Here's how the part is built. I have some questions about the finished solid (model axes, mm). Face numbers are marked on the shaded views. A direction names the side the tool comes from. Round coordinates to 2 decimals unless told otherwise and drop trailing zeros. Order: outer loops, then holes, each group sorted by start corner. A loop starts at its lowest first (then second) coordinate and runs counter-clockwise, first axis right, second up.
```python
from build123d import *

# Parameters (mm, degrees)
BOSS_EXTRUDE1_DEPTH             = 10
SKETCH5_W                       = 22
SKETCH5_H                       = 7
CUT_EXTRUDE2_DEPTH              = 28.349588662
FILLET3_R                       = 0.5
M3X0_5_TAPPED_HOLE1_D           = 2.5
M3X0_5_TAPPED_HOLE1_CSINK_D     = 3.05
M3X0_5_TAPPED_HOLE1_CSINK_ANGLE = 90
M8X1_0_TAPPED_HOLE1_D           = 7
M8X1_0_TAPPED_HOLE1_CSINK_D     = 8.05
M8X1_0_TAPPED_HOLE1_CSINK_ANGLE = 90


with BuildPart() as part:
    # Sketch1 → Boss-Extrude1 (new body)
    with BuildSketch(Plane.XY):
        with BuildLine():
            Line((-14, 9.141740125), (14, 9.141740125))
            ThreePointArc((14, 9.141740125), (16.828427125, 7.97016725), (18, 5.141740125))
            Line((18, 5.141740125), (18, -4.858259875))
            ThreePointArc((18, -4.858259875), (16.828427125, -7.686686999), (14, -8.858259875))
            Line((14, -8.858259875), (-14, -8.858259875))
            ThreePointArc((-14, -8.858259875), (-16.828427125, -7.686686999), (-18, -4.858259875))
            Line((-18, -4.858259875), (-18, 5.141740125))
            ThreePointArc((-18, 5.141740125), (-16.828427125, 7.97016725), (-14, 9.141740125))
        make_face()
    extrude(amount=BOSS_EXTRUDE1_DEPTH)

    # Sketch5 → Cut-Extrude2 (cut, through all)
    with BuildSketch(Plane(origin=(0, 9.141740125, 0), x_dir=(1, 0, 0), z_dir=(0, 1, 0))):
        Rectangle(SKETCH5_W, SKETCH5_H)
    extrude(amount=-CUT_EXTRUDE2_DEPTH, mode=Mode.SUBTRACT)

    # Fillet3
    fillet3_edges = [part.edges().sort_by_distance(p)[0] for p in [
        (-16.828427125, 7.97016725, 10),
        (-18, 0.141740125, 10),
        (-16.828427125, -7.686686999, 10),
        (0, -8.858259875, 10),
        (16.828427125, -7.686686999, 10),
        (11, -8.858259875, 1.75),
        (18, 0.141740125, 10),
        (0, -8.858259875, 3.5),
        (11, 0.141740125, 3.5),
        (-11, -8.858259875, 1.75),
        (-11, 0.141740125, 3.5),
        (-11, 9.141740125, 1.75),
        (0, 9.141740125, 3.5),
        (11, 9.141740125, 1.75),
        (16.828427125, 7.97016725, 10),
        (0, 9.141740125, 10),
    ]]
    fillet(fillet3_edges, radius=FILLET3_R)

    # M3x0.5 Tapped Hole1 (through all)
    with Locations(Plane(origin=(-13.335, 0.141740125, 10), x_dir=(1, 0, 0), z_dir=(0, 0, 1))):
        with Locations((0, 0), (26.67, 0)):
            CounterSinkHole(M3X0_5_TAPPED_HOLE1_D / 2, M3X0_5_TAPPED_HOLE1_CSINK_D / 2, counter_sink_angle=M3X0_5_TAPPED_HOLE1_CSINK_ANGLE)

    # M8x1.0 Tapped Hole1 (through all)
    with Locations(Plane(origin=(0, 0.141740125, 10), x_dir=(1, 0, 0), z_dir=(0, 0, 1))):
        with Locations((0, 0)):
            CounterSinkHole(M8X1_0_TAPPED_HOLE1_D / 2, M8X1_0_TAPPED_HOLE1_CSINK_D / 2, counter_sink_angle=M8X1_0_TAPPED_HOLE1_CSINK_ANGLE)


solid = part.part
```
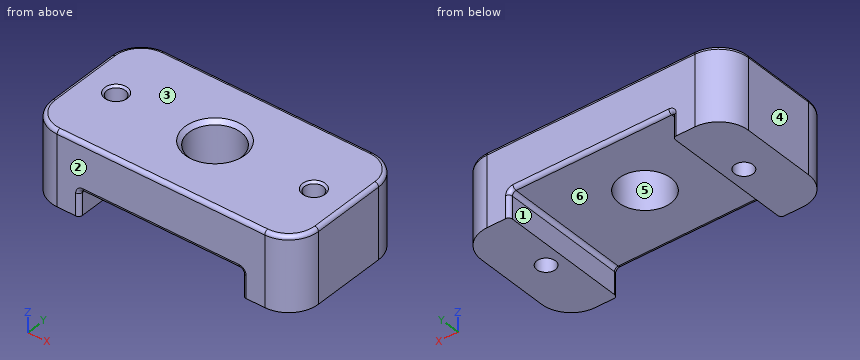
1) We'd pull the mould along X, two halves only. Please class the marked faces 3, 4, 5 and 6: +X half, -X half, draft (parallel to the pull), parting line (faces both ways), or undercut.
2) I'm going to push flat-ended pins straight in: pin 1 (4 mm diameter, centred on x = -2, z = 3, fed in from -Y); pin 2 (4 mm diameter, centred on x = 6.5, y = 7, fed in from -Z); pin 3 (3 mm diameter, centred on y = -7, z = 2.5, fed in from -X); pin 4 (2 mm diameter, centred on y = -6, z = 6, fed in from +X). Where does each tip first touch, or does it pass through?
3) If we section it at B-B (z = 1.5): Write out the boundary of the cut face in (x, y) (3 decimals).
4) I need wall thicknesses on line 1 (X direction, y = 0.25, z = 4.75); line 2 (Y direction, x = 0, z = 5.85); line 3 (Z direction, x = 2, y = -4.5). Which ranges of each line are inside material? Lowest first, please.
5) If we section it at D-D (z = 6.25): Write out the boundary of the cut face in (x, y) (3 decimals).
6) If we section it at A-A (x = 0): Write out the boundary of the cut face in (y, z) (3 decimals), plus the area to 3 significant figures.
7) If we section it at C-C (x = -5): Write out the boundary of the cut face in (y, z).
8) For the marked faces 1 and 2, which set-ups out of +Z, -Z, +X, -X, +Y, -Y let a thin tool reach every point of the face, with its end or its side?
Solutions:
1. face 3: draft
1. face 4: -X half
1. face 5: undercut
1. face 6: undercut
2. pin 1: stops at y = -8.86
2. pin 2: stops at z = 3.5
2. pin 3: stops at x = -17.95
2. pin 4: stops at x = 18
3. outline: (-18, -4.858) arc R4 ccw to (-14, -8.858) - (-11.5, -8.858) arc R0.5 ccw to (-11, -8.358) - (-11, 8.642) arc R0.5 ccw to (-11.5, 9.142) - (-14, 9.142) arc R4 ccw to (-18, 5.142) - close; (11, -8.358) arc R0.5 ccw to (11.5, -8.858) - (14, -8.858) arc R4 ccw to (18, -4.858) - (18, 5.142) arc R4 ccw to (14, 9.142) - (11.5, 9.142) arc R0.5 ccw to (11, 8.642) - close; hole circle Ø2.5 at (-13.335, 0.142); hole circle Ø2.5 at (13.335, 0.142)
4. line 1: x = -18 to -14.58, -12.09 to -3.5, 3.5 to 12.09, 14.58 to 18
4. line 2: y = -8.86 to -3.36, 3.64 to 9.14
4. line 3: z = 3.5 to 10
5. outline: (-18, -4.858) arc R4 ccw to (-14, -8.858) - (14, -8.858) arc R4 ccw to (18, -4.858) - (18, 5.142) arc R4 ccw to (14, 9.142) - (-14, 9.142) arc R4 ccw to (-18, 5.142) - close; hole circle Ø2.5 at (-13.335, 0.142); hole circle Ø7 at (0, 0.142); hole circle Ø2.5 at (13.335, 0.142)
6. outline: (-8.858, 4) arc R0.5 ccw to (-8.358, 3.5) - (-3.358, 3.5) - (-3.358, 9.475) - (-3.883, 10) - (-8.358, 10) arc R0.5 ccw to (-8.858, 9.5) - close; (3.642, 3.5) - (8.642, 3.5) arc R0.5 ccw to (9.142, 4) - (9.142, 9.5) arc R0.5 ccw to (8.642, 10) - (4.167, 10) - (3.642, 9.475) - close
6. area: 71.0 mm2
7. outline: (-8.86, 4) arc R0.5 ccw to (-8.36, 3.5) - (8.64, 3.5) arc R0.5 ccw to (9.14, 4) - (9.14, 9.5) arc R0.5 ccw to (8.64, 10) - (-8.36, 10) arc R0.5 ccw to (-8.86, 9.5) - close
8. face 1: -Z, +Y, -Y
8. face 2: +Z, -Z, +X, -X, -Y
